Check sheet for the drawn part. Datum: minimum x, y, z corner. Units: mm. A direction names the side the tool comes from. Round coordinates to 2 decimals unless told otherwise and drop trailing zeros. Write each loop counter-clockwise with the first axis right and the second up, starting at its lowest first coordinate (ties: lowest second). Pieces come first, ordered by that corner, then holes. Notation, with made-up numbers: M 22.25,88 L 54.25,88 A35 ccw 54.25,124 Z; hole C 84.25,70 d9. An arc over 180 degrees is marked long. Use a Markdown table: item, result.
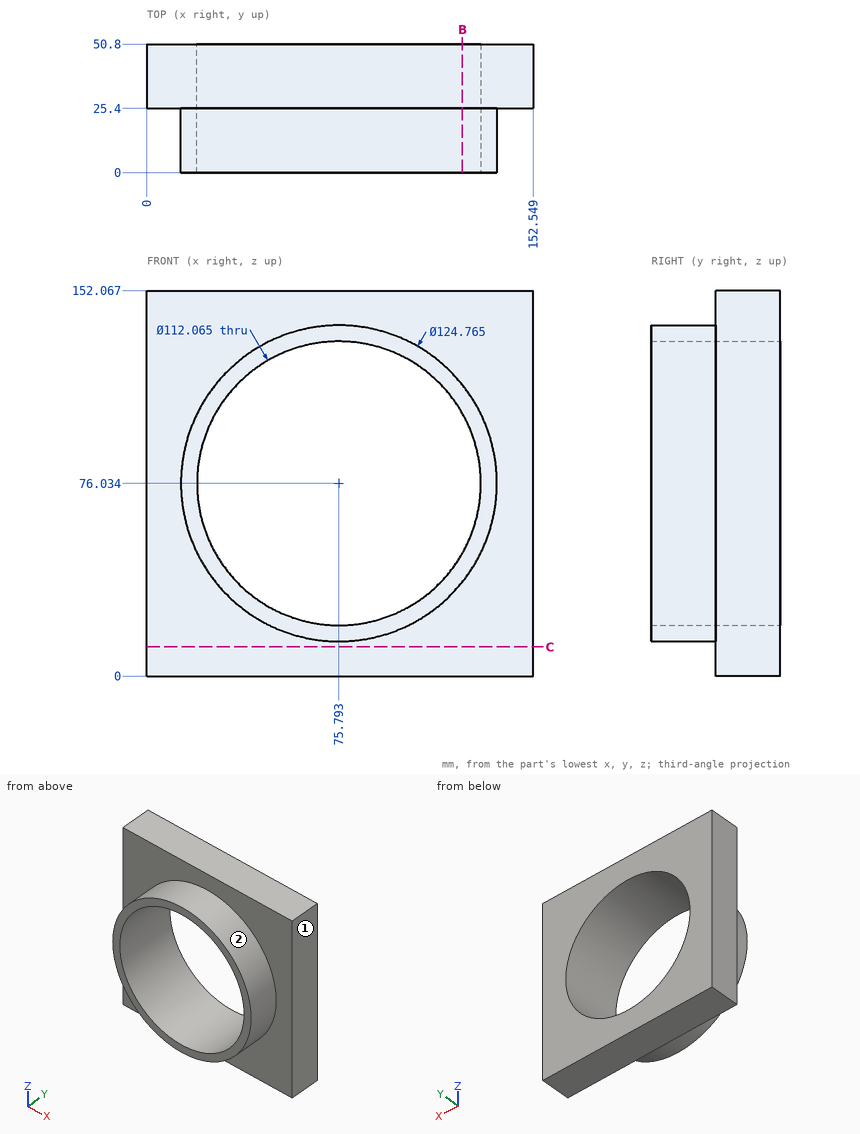
Item 1: Cross-section at B-B, the plane x = 124.5. Record the cut outline in (y, z) (1 decimal).
Outcome:
| item | result |
|---|---|
| outline | M 0,37.1 L 25.4,37.1 L 25.4,0 L 50.8,0 L 50.8,48.3 L 0,48.3 Z; M 0,103.7 L 50.8,103.7 L 50.8,152.1 L 25.4,152.1 L 25.4,115 L 0,115 Z |
Item 2: Access from +Z, -Z, +X, -X, +Y, -Y to the whole of each face (thin tool, end or side, straight path). Record for the marked faces 1 and 2.
Outcome:
| item | result |
|---|---|
| face 1 | +Z, -Z, +X, +Y, -Y |
| face 2 | -Y |
Item 3: Cross-section at C-C, the plane z = 11.5. Record the cut outline in (x, y).
Outcome:
| item | result |
|---|---|
| outline | M 0,25.4 L 152.55,25.4 L 152.55,50.8 L 0,50.8 Z |
Item 4: Material ranges on line 1 along Y through (x, z) = (141, 122); line 2 along X through (y, z) = (6.5, 33) (1 decimal); line 3 along Z through (x, y) = (125, 22) (1 decimal), recorded low to high. Write a range as from..to.
Outcome:
| item | result |
|---|---|
| line 1 | y = 25.4..50.8 |
| line 2 | x = 30.6..39.9, 111.7..121 |
| line 3 | z = 37.7..49.2, 102.8..114.4 |
Item 5: Go/stop test with flat-tipped pins: pin 1 (2 mm diameter, centred on y = 12, z = 60, fed in from -X); pin 2 (8 mm diameter, centred on x = 70, y = 19.5, fed in from +Z). Record where each tip stops, or that it passes through.
Outcome:
| item | result |
|---|---|
| pin 1 | stops at x = 15.25 |
| pin 2 | stops at z = 138.39 |
